Part print with two shaded views. Sizes in mm from the minimum x, y, z corner. Coordinates: 2 decimals unless noted, no trailing zeros. Order: outer loops, then holes, each group sorted by start corner. A loop starts at its lowest first (then second) coordinate and runs counter-clockwise, first axis right, second up.
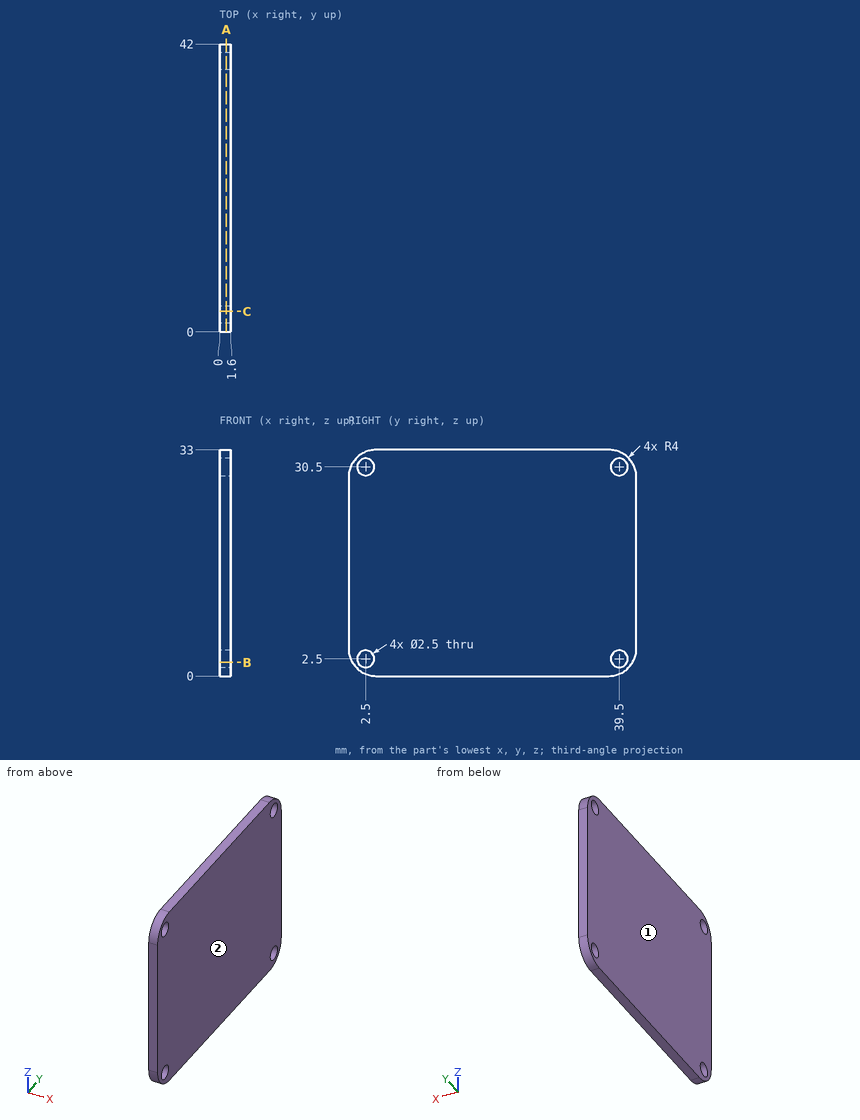
Q1. Cut at A-A on x = 1. Write the cut outline in (y, z).
Results list:
outline: (0, 4) arc R4 ccw to (4, 0) - (38, 0) arc R4 ccw to (42, 4) - (42, 29) arc R4 ccw to (38, 33) - (4, 33) arc R4 ccw to (0, 29) - close; hole circle Ø2.5 at (2.5, 2.5); hole circle Ø2.5 at (2.5, 30.5); hole circle Ø2.5 at (39.5, 2.5); hole circle Ø2.5 at (39.5, 30.5)
Q2. Wall check: line 1 along Y through (x, z) = (1.3, 30.5); line 2 along Z through (x, y) = (0.9, 39.5). Give the ranges that are in metal, low to high.
Results list:
line 1: y = 0.29 to 1.25, 3.75 to 38.25, 40.75 to 41.71
line 2: z = 0.29 to 1.25, 3.75 to 29.25, 31.75 to 32.71
Q3. Cut at B-B on z = 2. Write the cut outline in (x, y).
Results list:
outline: (0, 0.54) - (1.6, 0.54) - (1.6, 1.35) - (0, 1.35) - close; (0, 3.65) - (1.6, 3.65) - (1.6, 38.35) - (0, 38.35) - close; (0, 40.65) - (1.6, 40.65) - (1.6, 41.46) - (0, 41.46) - close
Q4. Mould opens along X. For the marked faces 1 and 2 say: pulls with the +X half, pulls with the -X half, needs draft (parallel to the pull), parting line crosses it, or undercut.
Results list:
face 1: pulls with the -X half
face 2: pulls with the +X half
Q5. Cut at C-C on y = 3. Write the cut outline in (x, z).
Results list:
outline: (0, 0.13) - (1.6, 0.13) - (1.6, 1.35) - (0, 1.35) - close; (0, 3.65) - (1.6, 3.65) - (1.6, 29.35) - (0, 29.35) - close; (0, 31.65) - (1.6, 31.65) - (1.6, 32.87) - (0, 32.87) - close
